Check sheet for the modelled part. Datum: model origin and axes. Units: mm. Round coordinates to 2 decimals unless told otherwise and drop trailing zeros. Order: outer loops, then holes, each group sorted by start corner. A loop starts at its lowest first (then second) coordinate and runs counter-clockwise, first axis right, second up.
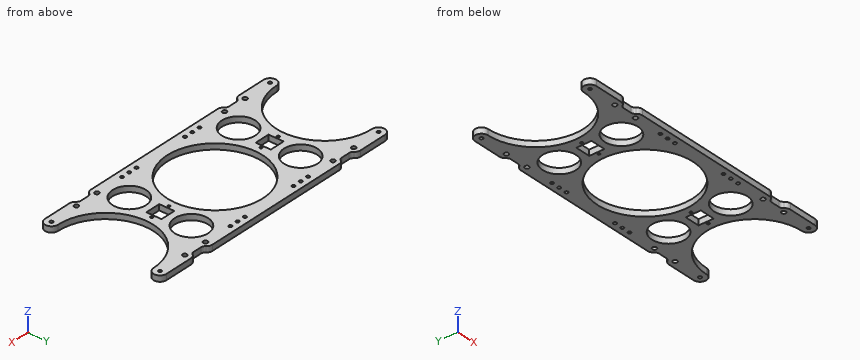
from build123d import *

# Parameters (mm, degrees)
SKETCH1_R            = 83.05
SKETCH1_R_2          = 29.075
SKETCH1_R_3          = 2.2
SKETCH1_R_4          = 3.75
SKETCH1_W            = 26.4
SKETCH1_H            = 26.4
BOSS_EXTRUDE1_DEPTH  = 5
M5_CLEARANCE_HOLE1_D = 5.5
FILLET1_R            = 10


with BuildPart() as part:
    # Sketch1 → Boss-Extrude1 (new body, symmetric)
    with BuildSketch(Plane.XY):
        with BuildLine():
            Line((-225.104242519, 105.55), (-167.604242519, 105.55))
            ThreePointArc((-167.604242519, 105.55), (-165.407543378, 100.246699141), (-160.104242519, 98.05))
            Line((-160.104242519, 98.05), (-145.104242519, 98.05))
            ThreePointArc((-145.104242519, 98.05), (-139.80094166, 100.246699141), (-137.604242519, 105.55))
            Line((-137.604242519, 105.55), (137.604242519, 105.55))
            ThreePointArc((137.604242519, 105.55), (139.80094166, 100.246699141), (145.104242519, 98.05))
            Line((145.104242519, 98.05), (160.104242519, 98.05))
            ThreePointArc((160.104242519, 98.05), (165.407543378, 100.246699141), (167.604242519, 105.55))
            Line((167.604242519, 105.55), (225.104242519, 105.55))
            ThreePointArc((225.104242519, 105.55), (236.354242519, 94.3), (225.104242519, 83.05))
            ThreePointArc((225.104242519, 83.05), (142.054242519, 0), (225.104242519, -83.05))
            ThreePointArc((225.104242519, -83.05), (236.354242519, -94.3), (225.104242519, -105.55))
            Line((225.104242519, -105.55), (167.604242519, -105.55))
            ThreePointArc((167.604242519, -105.55), (165.407543378, -100.246699141), (160.104242519, -98.05))
            Line((160.104242519, -98.05), (145.104242519, -98.05))
            ThreePointArc((145.104242519, -98.05), (139.80094166, -100.246699141), (137.604242519, -105.55))
            Line((137.604242519, -105.55), (-137.604242519, -105.55))
            ThreePointArc((-137.604242519, -105.55), (-139.80094166, -100.246699141), (-145.104242519, -98.05))
            Line((-145.104242519, -98.05), (-160.104242519, -98.05))
            ThreePointArc((-160.104242519, -98.05), (-165.407543378, -100.246699141), (-167.604242519, -105.55))
            Line((-167.604242519, -105.55), (-225.104242519, -105.55))
            ThreePointArc((-225.104242519, -105.55), (-236.354242519, -94.3), (-225.104242519, -83.05))
            ThreePointArc((-225.104242519, -83.05), (-142.054242519, 0), (-225.104242519, 83.05))
            ThreePointArc((-225.104242519, 83.05), (-236.354242519, 94.3), (-225.104242519, 105.55))
        make_face()
        Circle(SKETCH1_R, mode=Mode.SUBTRACT)
        with Locations((112.552121259, 53.975)):
            Circle(SKETCH1_R_2, mode=Mode.SUBTRACT)
        with Locations((112.552121259, -53.975)):
            Circle(SKETCH1_R_2, mode=Mode.SUBTRACT)
        with Locations((-112.552121259, -53.975)):
            Circle(SKETCH1_R_2, mode=Mode.SUBTRACT)
        with Locations((-112.552121259, 53.975)):
            Circle(SKETCH1_R_2, mode=Mode.SUBTRACT)
        with Locations((94.852121259, 0)):
            Circle(SKETCH1_R_3, mode=Mode.SUBTRACT)
        with Locations((130.252121259, 0)):
            Circle(SKETCH1_R_3, mode=Mode.SUBTRACT)
        with Locations((-130.252121259, 0)):
            Circle(SKETCH1_R_3, mode=Mode.SUBTRACT)
        with Locations((-94.852121259, 0)):
            Circle(SKETCH1_R_3, mode=Mode.SUBTRACT)
        with Locations((-173.854242519, 94.3)):
            Circle(SKETCH1_R_4, mode=Mode.SUBTRACT)
        with Locations((-131.354242519, 94.3)):
            Circle(SKETCH1_R_4, mode=Mode.SUBTRACT)
        with Locations((-131.354242519, -94.3)):
            Circle(SKETCH1_R_4, mode=Mode.SUBTRACT)
        with Locations((-173.854242519, -94.3)):
            Circle(SKETCH1_R_4, mode=Mode.SUBTRACT)
        with Locations((131.354242519, -94.3)):
            Circle(SKETCH1_R_4, mode=Mode.SUBTRACT)
        with Locations((173.854242519, -94.3)):
            Circle(SKETCH1_R_4, mode=Mode.SUBTRACT)
        with Locations((131.354242519, 94.3)):
            Circle(SKETCH1_R_4, mode=Mode.SUBTRACT)
        with Locations((173.854242519, 94.3)):
            Circle(SKETCH1_R_4, mode=Mode.SUBTRACT)
        with Locations((-112.552121259, 0)):
            Rectangle(SKETCH1_W, SKETCH1_H, mode=Mode.SUBTRACT)
        with Locations((112.552121259, 0)):
            Rectangle(SKETCH1_W, SKETCH1_H, mode=Mode.SUBTRACT)
    extrude(amount=BOSS_EXTRUDE1_DEPTH, both=True)

    # M5 Clearance Hole1 (through all)
    with Locations(Plane.XY.offset(5)):
        with Locations((-80, 94.3), (-65, 94.3), (-50, 94.3), (50, 94.3), (65, 94.3), (80, 94.3), (-80, -94.3), (-65, -94.3), (-50, -94.3), (50, -94.3), (65, -94.3), (80, -94.3), (0, 0), (-225.104242519, 94.3), (225.104242519, 94.3), (225.104242519, -94.3), (-225.104242519, -94.3)):
            Hole(M5_CLEARANCE_HOLE1_D / 2)

    # Fillet1
    fillet1_edges = [part.edges().sort_by_distance(p)[0] for p in [
        (167.604242519, -105.55, 0),
        (137.604242519, -105.55, 0),
        (-137.604242519, -105.55, 0),
        (-167.604242519, -105.55, 0),
        (-167.604242519, 105.55, 0),
        (-137.604242519, 105.55, 0),
        (137.604242519, 105.55, 0),
        (167.604242519, 105.55, 0),
    ]]
    fillet(fillet1_edges, radius=FILLET1_R)


solid = part.part
1) Sectioned sample at A-A on x = 0. Record the cut outline in (y, z), and give its area (3 significant figures).
2) Sectioned sample at B-B on y = -73.5. Record the cut outline in (x, z), and give its area (3 significant figures).
3) Sectioned sample at C-C on y = 8.5. Record the cut outline in (x, z).
4) Gauge pin test, flat ends, axial feed: pin 1 (9 mm diameter, centred on x = -80, y = -94.3, fed in from +Z); pin 2 (1 mm diameter, centred on y = 14.5, z = 3, fed in from -X); pin 3 (2 mm diameter, centred on y = 1, z = 2, fed in from +X); pin 4 (6 mm diameter, centred on y = -40, z = 1, fed in from +X). Record the tip position at first contact, or that the pin passes through.
5) Sectioned sample at D-D on x = 198. Record the cut outline in (y, z), and give its area (3 significant figures).
6) Scan lines: line 1 (X direction, y = 54.5, z = -3.75); line 2 (X direction, y = -5, z = -1.5); line 3 (Y direction, x = 50, z = -1). Record each from-to range of solid material in increasing order.
Values found:
1. outline: (-105.55, -5) - (-83.05, -5) - (-83.05, 5) - (-105.55, 5) - close; (83.05, -5) - (105.55, -5) - (105.55, 5) - (83.05, 5) - close
1. area: 450 mm2
2. outline: (-186.44, -5) - (-134.1, -5) - (-134.1, 5) - (-186.44, 5) - close; (-91.01, -5) - (-38.67, -5) - (-38.67, 5) - (-91.01, 5) - close; (38.67, -5) - (91.01, -5) - (91.01, 5) - (38.67, 5) - close; (134.1, -5) - (186.44, -5) - (186.44, 5) - (134.1, 5) - close
2. area: 2,090 mm2
3. outline: (-142.49, -5) - (-125.75, -5) - (-125.75, 5) - (-142.49, 5) - close; (-99.35, -5) - (-82.61, -5) - (-82.61, 5) - (-99.35, 5) - close; (82.61, -5) - (99.35, -5) - (99.35, 5) - (82.61, 5) - close; (125.75, -5) - (142.49, -5) - (142.49, 5) - (125.75, 5) - close
4. pin 1: stops at z = 5
4. pin 2: stops at x = -143.42
4. pin 3: stops at x = 142.08
4. pin 4: stops at x = 154.05
5. outline: (-105.55, -5) - (-78.5, -5) - (-78.5, 5) - (-105.55, 5) - close; (78.5, -5) - (105.55, -5) - (105.55, 5) - (78.5, 5) - close
5. area: 541 mm2
6. line 1: x = -162.44 to -141.62, -83.48 to -62.67, 62.67 to 83.48, 141.62 to 162.44
6. line 2: x = -142.2 to -125.75, -99.35 to -82.9, 82.9 to 99.35, 125.75 to 142.2
6. line 3: y = -105.55 to -97.05, -91.55 to -66.31, 66.31 to 91.55, 97.05 to 105.55
